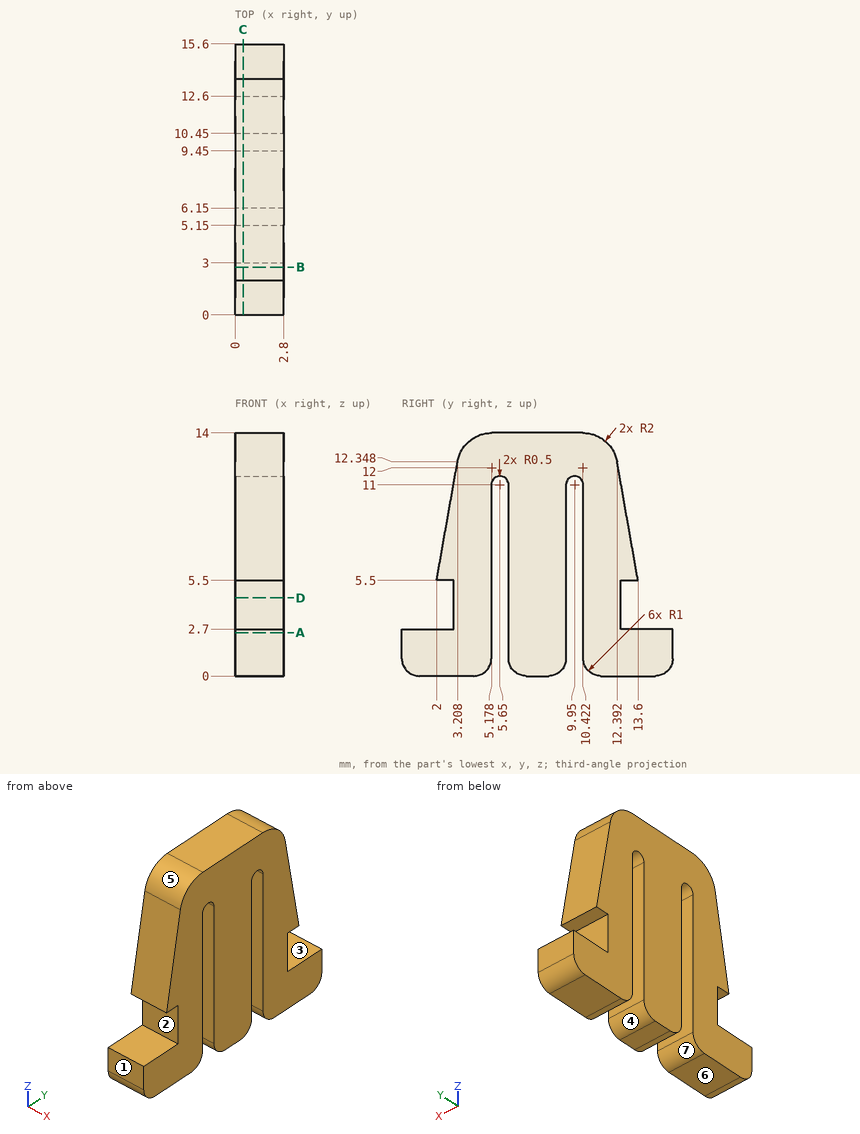
Job drawing, mm, ordinate dimensions from the low corner. One solid piece. A direction names the side the tool comes from. Round coordinates to 2 decimals unless told otherwise and drop trailing zeros. Loops run counter-clockwise (first coordinate to the right, second up) from the corner with the lowest first, then second, coordinate; pieces in that order, holes last.
Item 1: 3-axis set-ups, long thin cutter, end or side, ignore diameter. For the marked faces 1, 2 and 3: which of +Z, -Z, +X, -X, +Y, -Y reach the whole face in a straight line?
Item 2: Cut at B-B, the plane y = 2.75. Give the cut face in (x, z).
Item 3: Drill centre lines: line 1 (Y direction, x = 1.8, z = 4.25); line 2 (Y direction, x = 0.7, z = 1); line 3 (Z direction, x = 0.65, y = 1.75). Where is each one in solid material? Low to high.
Item 4: Cut at C-C, the plane x = 0.45. Give the cut face in (y, z).
Item 5: Drop flat-ended pins along their axis: P1, Ø1.4, axis at x = 1.5, z = 5, coming from the +Y side; P2, Ø1.4, axis at x = 0.5, z = 3.5, coming from the -Y side; P3, Ø1.4, axis at x = 2, z = 6.5, coming from the +Y side. Give the stop position or say it passes through.
Item 6: Mould opens along Y. For the marked faces 4, 5, 6 and 7 say: +Y half, -Y half, draft (parallel to the pull), parting line (faces both ways), or undercut.
Item 7: Cut at D-D, the plane z = 4.5. Give the cut face in (x, y), then the cut area to 3 significant figures.
Item 8: Cut at A-A, the plane z = 2.5. Give the cut face in (x, y).
A:
1. face 1: +Z, -Z, +X, -X, -Y
1. face 2: +X, -X, -Y
1. face 3: +X, -X, +Y
2. outline: (0, 0) - (2.8, 0) - (2.8, 2.7) - (0, 2.7) - close; (0, 5.5) - (2.8, 5.5) - (2.8, 9.75) - (0, 9.75) - close
3. line 1: y = 3 to 5.15, 6.15 to 9.45, 10.45 to 12.6
3. line 2: y = 0 to 5.15, 6.15 to 9.45, 10.45 to 15.6
3. line 3: z = 0 to 2.7
4. outline: (0, 1) arc R1 ccw to (1, 0) - (4.15, 0) arc R1 ccw to (5.15, 1) - (5.15, 11) arc R0.5 cw to (6.15, 11) - (6.15, 1) arc R1 ccw to (7.15, 0) - (8.45, 0) arc R1 ccw to (9.45, 1) - (9.45, 11) arc R0.5 cw to (10.45, 11) - (10.45, 1) arc R1 ccw to (11.45, 0) - (14.6, 0) arc R1 ccw to (15.6, 1) - (15.6, 2.7) - (12.6, 2.7) - (12.6, 5.5) - (13.6, 5.5) - (12.39, 12.35) arc R2 ccw to (10.42, 14) - (5.18, 14) arc R2 ccw to (3.21, 12.35) - (2, 5.5) - (3, 5.5) - (3, 2.7) - (0, 2.7) - close
5. P1: stops at y = 13.6
5. P2: stops at y = 3
5. P3: stops at y = 13.55
6. face 4: undercut
6. face 5: -Y half
6. face 6: draft
6. face 7: undercut
7. outline: (0, 3) - (2.8, 3) - (2.8, 5.15) - (0, 5.15) - close; (0, 6.15) - (2.8, 6.15) - (2.8, 9.45) - (0, 9.45) - close; (0, 10.45) - (2.8, 10.45) - (2.8, 12.6) - (0, 12.6) - close
7. area: 21.3 mm2
8. outline: (0, 0) - (2.8, 0) - (2.8, 5.15) - (0, 5.15) - close; (0, 6.15) - (2.8, 6.15) - (2.8, 9.45) - (0, 9.45) - close; (0, 10.45) - (2.8, 10.45) - (2.8, 15.6) - (0, 15.6) - close
